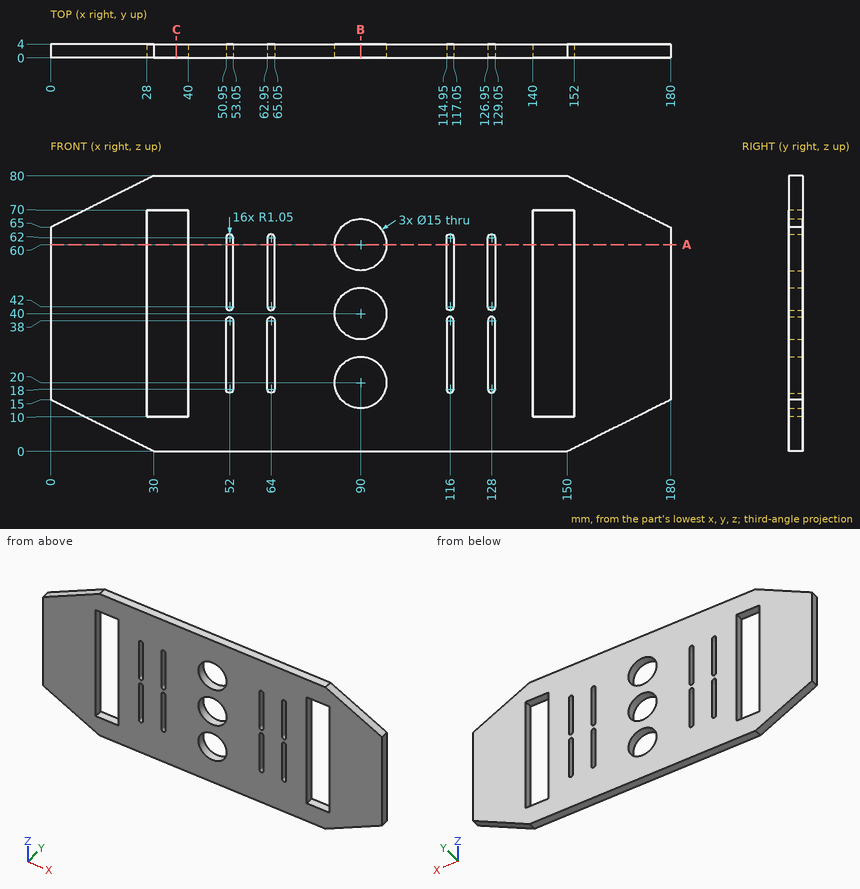
Here's the drawing with two shaded views (mm, measured from the low corner). I have some questions. Give positions to 0.01 mm unless a question says otherwise; leave off trailing zeros. Loops run counter-clockwise (first coordinate to the right, second up) from the corner with the lowest first, then second, coordinate; pieces in that order, holes last. Notation, with made-up numbers: M 28,4 L 66,4 A32 ccw 66,32 Z; hole C 30.25,21.25 d5. An arc over 180 degrees is marked long. Use one line per item in the form item = value. Start each with the question number.
Q1. If we section it at C-C (x = 36.5): Write out the boundary of the cut face in (y, z), then the cut area to 3 significant figures.
Q2. I need wall thicknesses on line 1 along Z through (x, y) = (90, 3.1); line 2 along Z through (x, y) = (128, 2.4); line 3 along X through (y, z) = (2.9, 40). Which ranges of each line are inside material? Lowest first, please.
Q3. If we section it at A-A (z = 60): State how many separate pieces and enclosed holes the cut face has, then the cut area to 3 significant figures.
Q4. Will this pin go through, and if not, where does the flat tip stop? pin 1 Ø9 at (x, z) = (90, 60) entering from -Y.
Q5. If we section it at B-B (x = 90): Write out the boundary of the cut face in (y, z), then the cut area to 3 significant figures.
Taken from the geometry:
q1.outline = M 0,0 L 4,0 L 4,10 L 0,10 Z; M 0,70 L 4,70 L 4,80 L 0,80 Z
q1.area = 80.0 mm^2
q2.line_1 = 0 to 12.5, 27.5 to 32.5, 47.5 to 52.5, 67.5 to 80
q2.line_2 = 0 to 16.95, 39.05 to 40.95, 63.05 to 80
q2.line_3 = 0 to 28, 40 to 82.5, 97.5 to 140, 152 to 180
q3.separate_pieces = 8
q3.enclosed_holes = 0
q3.area = 530 mm^2
q4.pin_1 = through
q5.outline = M 0,0 L 4,0 L 4,12.5 L 0,12.5 Z; M 0,27.5 L 4,27.5 L 4,32.5 L 0,32.5 Z; M 0,47.5 L 4,47.5 L 4,52.5 L 0,52.5 Z; M 0,67.5 L 4,67.5 L 4,80 L 0,80 Z
q5.area = 140 mm^2
